Read the model definition and answer for the solid it produces. Units are mm, in the model's axes. A direction names the side the tool comes from. Give positions to 0.01 mm unless a question says otherwise; leave off trailing zeros. Loops run counter-clockwise (first coordinate to the right, second up) from the corner with the lowest first, then second, coordinate; pieces in that order, holes last. Notation, with made-up numbers: (47.5, -7.75) -> (58.5, -7.75) arc R22 ccw to (58.5, 1.25) -> close; hole circle Ø1 at (2, 39.25). An arc over 180 degrees is marked (long way). Write each question's results on one line, items separated by ' | '. Start each with the question number.
Item 1: Determine the mould class of faces 4 (the flat face through (3, 0, 28)), 5 (the flat face through (3, -165.1, 20)), 6 (the cylindrical face through (2.82, -82.43, 12.79)), 7 (the flat face through (3, -63, 55.88)) for opening direction Y: +Y half, -Y half, draft (parallel to the pull), parting line (faces both ways), or undercut.
Item 2: Section D-D on x = 1.7 is taken. State how many separate pieces and enclosed holes the cut face has, and give its area (3 significant figures).
Item 3: Each of these flat-tipped pins is pushed along its axis until it touches: P1, Ø1.5, axis at x = 3.5, y = -127.5, coming from the -Z side; P2, Ø6.5, axis at y = -133.35, z = 24.13, coming from the +X side. Where does it stop, or does it pass through?
Item 4: Section A-A on z = 12.7 is taken. Write down the section's boundary in (x, y) (3 decimals), and give its area (3 significant figures).
Item 5: Section C-C on z = 24.13 is taken. Write down the section's boundary in (x, y) (1 decimal).
Item 6: Which of the six approach directions +Z, -Z, +X, -X, +Y, -Y give full straight-line access (tool end or side, diameter ignored) to faces 1 (the flat face through (3, -84, 0)), 2 (the flat face through (3, -93, 16.669)), 3 (the flat face through (3, -126.938, 48))?
Item 7: Section B-B on y = -133.35 is taken. Write down the section's boundary in (x, z) (3 decimals).
Item 8: Find the intervals of material crossed by line 1 (Y direction, x = 5.15, z = 48); line 2 (Z direction, x = 4.9, y = -92.5); line 3 (Y direction, x = 0.35, z = 13), in increasing order.
```python
from build123d import *

# Parameters (mm, degrees)
SKETCH1_R             = 3.9751
SKETCH1_R_2           = 14.249999948
BOSS_EXTRUDE1_DEPTH   = 5.715
M4X0_7_TAPPED_HOLE1_D = 3.3
CHAMFER1_SIZE         = 1.5367


with BuildPart() as part:
    # Sketch1 → Boss-Extrude1 (new body)
    with BuildSketch(Plane.YZ):
        Polygon((-165.1, 0), (0, 0), (0, 55.88), (-126.937814396, 55.88), (-126.937814396, 40.052578354), (-165.1, 40.052578354), align=None)
        with BuildLine():
            ThreePointArc((-99.098846149, 8.73125), (-103.067596149, 12.7), (-99.098846149, 16.66875))
            Line((-99.098846149, 16.66875), (-86.398846149, 16.66875))
            ThreePointArc((-86.398846149, 16.66875), (-82.430096149, 12.7), (-86.398846149, 8.73125))
            Line((-86.398846149, 8.73125), (-99.098846149, 8.73125))
        make_face(mode=Mode.SUBTRACT)
        with Locations(Location((-133.35, 24.13, 0), (0, 0, 270))):
            Circle(SKETCH1_R, mode=Mode.SUBTRACT)
        with Locations(Location((-31.9024, 24.13, 0), (0, 0, 270))):
            Circle(SKETCH1_R, mode=Mode.SUBTRACT)
        with Locations(Location((-86.398846149, 36.137660549, 0), (0, 0, 270))):
            Circle(SKETCH1_R_2, mode=Mode.SUBTRACT)
    extrude(amount=BOSS_EXTRUDE1_DEPTH)

    # M4x0.7 Tapped Hole1 (through all)
    with Locations(Plane(origin=(5.715, 0, 0), x_dir=(0, 0, -1), z_dir=(1, 0, 0))):
        with Locations((-48.158475855, -74.378030844), (-24.116845244, -74.378030844), (-24.116845244, -98.419661455), (-48.158475855, -98.419661455)):
            Hole(M4X0_7_TAPPED_HOLE1_D / 2)

    # Chamfer1
    chamfer1_edges = [part.edges().sort_by_distance(p)[0] for p in [
        (5.715, -31.9024, 28.1051),
        (5.715, -133.35, 28.1051),
    ]]
    chamfer(chamfer1_edges, length=CHAMFER1_SIZE)


solid = part.part
```
Findings:
1) face 4: +Y half | face 5: -Y half | face 6: undercut | face 7: draft
2) separate pieces: 1 | enclosed holes: 8 | area: 7,700 mm2
3) P1: z = 0 | P2: through
4) outline: (0, -165.1) -> (5.715, -165.1) -> (5.715, -103.068) -> (0, -103.068) -> close; (0, -82.43) -> (5.715, -82.43) -> (5.715, 0) -> (0, 0) -> close | area: 826 mm2
5) outline: (0, -165.1) -> (5.7, -165.1) -> (5.7, -138.9) -> (4.2, -137.3) -> (0, -137.3) -> close; (0, -129.4) -> (4.2, -129.4) -> (5.7, -127.8) -> (5.7, -100.1) -> (0, -100.1) -> close; (0, -96.8) -> (5.7, -96.8) -> (5.7, -94.1) -> (0, -94.1) -> close; (0, -78.7) -> (5.7, -78.7) -> (5.7, -76) -> (0, -76) -> close; (0, -72.7) -> (5.7, -72.7) -> (5.7, -37.4) -> (4.2, -35.9) -> (0, -35.9) -> close; (0, -27.9) -> (4.2, -27.9) -> (5.7, -26.4) -> (5.7, 0) -> (0, 0) -> close
6) face 1: -Z, +X, -X, +Y, -Y | face 2: +X, -X | face 3: +Z, +X, -X, -Y
7) outline: (0, 0) -> (5.715, 0) -> (5.715, 18.618) -> (4.178, 20.155) -> (0, 20.155) -> close; (0, 28.105) -> (4.178, 28.105) -> (5.715, 29.642) -> (5.715, 40.053) -> (0, 40.053) -> close
8) line 1: -126.94 to -100.06, -96.78 to -94.29, -78.5 to -76.02, -72.74 to 0 | line 2: 0 to 8.73, 16.67 to 23.26, 49.02 to 55.88 | line 3: -165.1 to -103.06, -82.44 to 0
